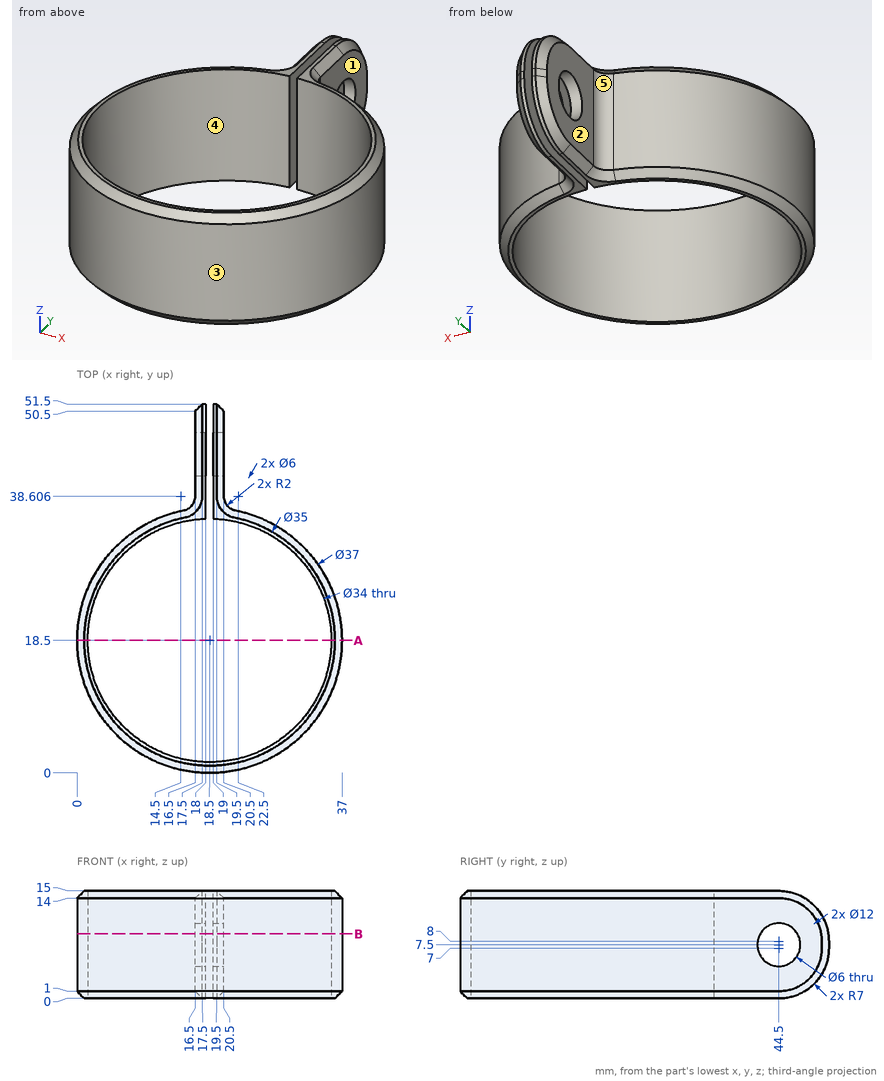
Could you check a few things on this drawing? It's one solid part, dimensions in mm from its lowest x, y, z. A direction names the side the tool comes from. Give positions to 0.01 mm unless a question says otherwise; leave off trailing zeros. Order: outer loops, then holes, each group sorted by start corner. A loop starts at its lowest first (then second) coordinate and runs counter-clockwise, first axis right, second up. Notation, with made-up numbers: (25, 17.25) - (47, 17.25) arc R14 ccw to (47, 32.25) - close; hole circle Ø4 at (-8.5, -32). An arc over 180 degrees is marked (long way). One line per item, written item: value. Start each with the question number.
1. For the marked faces 1 and 2, which set-ups out of +Z, -Z, +X, -X, +Y, -Y let a thin tool reach every point of the face, with its end or its side?
2. Thinking about a two-plate mould opening in Y: for the marked faces 3, 4 and 5, which applies, +Y half, -Y half, draft (parallel to the pull), parting line (faces both ways), or undercut?
3. If I drill on probe 1 along X at (y, z) = (41, 1.5); probe 2 along X at (y, z) = (5.5, 5.25); probe 3 along Y at (x, z) = (18.5, 7), over which ranges is the centre line in solid material (lowest first)?
4. Imagine slicing it at B-B on z = 9. Give the number of separate pieces and of enclosed holes in the cut face, plus the area to 3 significant figures.
5. Imagine slicing it at A-A on y = 18.5. List the corners of the cut face in (x, z) for me.
6. For P1, Ø8, axis at y = 44.5, z = 7.5, coming from the +X side; P2, Ø20.5, axis at x = 18.5, y = 18.5, coming from the +Z side; P3, Ø5, axis at y = 29, z = 2.5, coming from the +X side; P4, Ø8, axis at x = 13, z = 2, coming from the -Y side, each with a flat end and sliding along its axis, tell me the tip position at first contact or that it passes through.
Values:
1. face 1: +Z, -Z, +X, +Y
1. face 2: +Z, -Z, -X, +Y
2. face 3: parting line
2. face 4: undercut
2. face 5: +Y half
3. probe 1: 16.5 to 18, 19 to 20.5
3. probe 2: 5.34 to 7.55, 29.45 to 31.66
3. probe 3: 0 to 1.5
4. separate pieces: 3
4. enclosed holes: 0
4. area: 194 mm²
5. outline: (0, 1) - (1, 0) - (1.5, 0) - (1.5, 15) - (1, 15) - (0, 14) - close; (35.5, 0) - (36, 0) - (37, 1) - (37, 14) - (36, 15) - (35.5, 15) - close
6. P1: x = 20.5
6. P2: through
6. P3: x = 35.18
6. P4: y = 0.06
